Source: CAD feature listing. Evaluate the final solid. Frame: model axes, mm. A direction names the side the tool comes from. Round coordinates to 2 decimals unless told otherwise and drop trailing zeros. Order: outer loops, then holes, each group sorted by start corner. A loop starts at its lowest first (then second) coordinate and runs counter-clockwise, first axis right, second up. Notation, with made-up numbers: (34.5, 59) - (88.5, 59) arc R24 cw to (88.5, 82) - close; hole circle Ø2 at (-39, 18). An arc over 180 degrees is marked (long way). Use one line per item in the form item = value. Start each with the question number.
Q1. Pin query (flat end, axial travel): pin 1 Ø7 at (x, z) = (-0.5, 2) entering from +Y; pin 2 Ø6 at (x, y) = (5, 18) entering from -Z; pin 3 Ø4 at (y, z) = (33, -4.5) entering from -X. Return the tip coordinate at first contact, or that it passes through.
Q2. Cut plane A-A, the plane y = 65. Return the cut outline in (x, z).
Q3. Ray query, line 1 (Z direction, x = 0, y = 58); line 2 (Z direction, x = 0, y = -5.5); line 3 (Y direction, x = -6, z = 10.75). Return the intervals inside material, ascending. Write a range as [from, to].
Q4. Set-up query: faces 1 (the cylindrical face through (-7.964, 36.975, -2.508)), 2 (the flat face through (7.366, 75.74, -7.927)), 3 (the flat face through (0, 0, 0)). Return all of +Z, -Z, +X, -X, +Y, -Y with unobstructed straight access to the full face (end or side cutting, diameter ignored); none if empty.
Q5. Draft query along Z for faces 4 (the cylindrical face through (0, -7, 1)), 5 (the cylindrical face through (9.5, 75.7, 0)), 6 (the flat face through (-9, 75, 0)). Return one class per face: released by +Z, released by -Z, zero draft, split by the parting line, or undercut.
Autodesk Inventor part; units mm, degrees
ref_plane "YZ Plane" through (0, 0, 0) normal (1, 0, 0) x (0, 1, 0)
ref_plane "XZ Plane" through (0, 0, 0) normal (0, 1, 0) x (-1, 0, 0)
ref_plane "XY Plane" through (0, 0, 0) normal (0, 0, 1) x (1, 0, 0)
sketch "Sketch1" plane through (0, 0, 0) normal (0, 1, 0) x (-1, 0, 0)
  circle A0 centre (0, 0) radius 8.35
  circle A1 centre (0, 0) radius 7.1
  dimension "d0" = 16.7
  dimension "d1" = 14.2
extrude "Extrusion1" add sketch "Sketch1" along normal blind 75
sketch "Sketch2" plane through (0, 75, 0) normal (0, 1, 0) x (1, 0, 0)
  circle A0 centre (0, 0) radius 9.5
  circle A1 centre (0, 0) radius 7.1
  line L0 (9.5, -15) -> (-9.5, -15) construction
  line L1 (-9.5, -15) -> (-9.5, 15) construction
  line L2 (-9.5, 15) -> (9.5, 15) construction
  line L3 (9.5, 15) -> (9.5, -15) construction
  line L4 (9.5, -15) -> (-9.5, 15) construction
  line L5 (-9.5, -15) -> (9.5, 15) construction
  line L6 (5, 15) -> (-5, 15)
  line L7 (-5, 15) -> (-9.0094, 3.0135)
  line L8 (-9.0094, 3.0135) -> (9, 3.0414) construction
  line L9 (9, 3.0414) -> (5, 15)
  line L10 (0, 0) -> (-9.5, 0) construction
  line L11 (5, -15) -> (-5, -15)
  line L12 (-5, -15) -> (-9.0094, -3.0135)
  line L13 (9, -3.0414) -> (5, -15)
  point P0 (-9.0094, -3.0135)
  dimension "d4" = 14.2
  dimension "d5" = 19
  dimension "d6" = 30
  dimension "d7" = 5
  dimension "d8" = 5
extrude "Extrusion2" add sketch "Sketch2" along normal blind 1.5
sketch "Sketch3" plane through (0, 0, 0) normal (0, 0, 1) x (1, 0, 0)
  line L0 (8.35, 0) -> (-8.35, 0)
  line L1 (-8.35, 0) -> (-2.3, -2.7)
  line L2 (-2.3, -2.7) -> (0, -2.7)
  line L3 (0, -2.7) -> (0, 0) construction
  line L4 (-8.35, 0) -> (0, 0)
  line L5 (-5, 76.5) -> (5, 76.5)
  line L6 (-8.35, 0) -> (0, 0)
  line L7 (0, -2.7) -> (0, 0)
  line L8 (0, -18.54) -> (0, 92.34)
  dimension "d11" = 79.2
  dimension "d12" = 2.3
revolve "Revolution1" add sketch "Sketch3" angle 360 about axis through (0, 0, 0) along (0, 1, 0)
sketch "Sketch4" plane through (0, -2.7, 0) normal (0, -1, 0) x (1, 0, 0)
  circle A0 centre (0, 0) radius 2.3
  circle A1 centre (0, 0) radius 1
  circle A2 centre (0, 0) radius 2.3
  dimension "d14" = 2
extrude "Extrusion3" add sketch "Sketch4" along normal blind 9
chamfer "Chamfer1" distance 1 angle 45 1 edges at (-2.3, -11.7, 0)
fillet "Fillet1" radius 3 4 edges at (5, 75.75, -15) (5, 75.75, 15) (-5, 75.75, -15) (-5, 75.75, 15)
sketch "Sketch5" plane through (0, 75, 0) normal (0, -1, 0) x (1, 0, 0)
  circle A0 centre (0, 0) radius 8.7914
  circle A1 centre (0, 0) radius 2.3
  circle A2 centre (0, 0) radius 8.35
extrude "Extrusion4" [suppressed]
properties part number "10 mL syringe"
Completed:
q1.pin_1 = 0
q1.pin_2 = -8.11
q1.pin_3 = -7.97
q2.outline = circle Ø16.7 at (0, 0); hole circle Ø14.2 at (0, 0)
q3.line_1 = [-8.35, -7.1], [7.1, 8.35]
q3.line_2 = [-2.3, -1], [1, 2.3]
q3.line_3 = [75, 76.5]
q4.face_1 = -Y
q4.face_2 = -Z, +X, +Y, -Y
q4.face_3 = +Y
q5.face_4 = undercut
q5.face_5 = split by the parting line
q5.face_6 = zero draft
